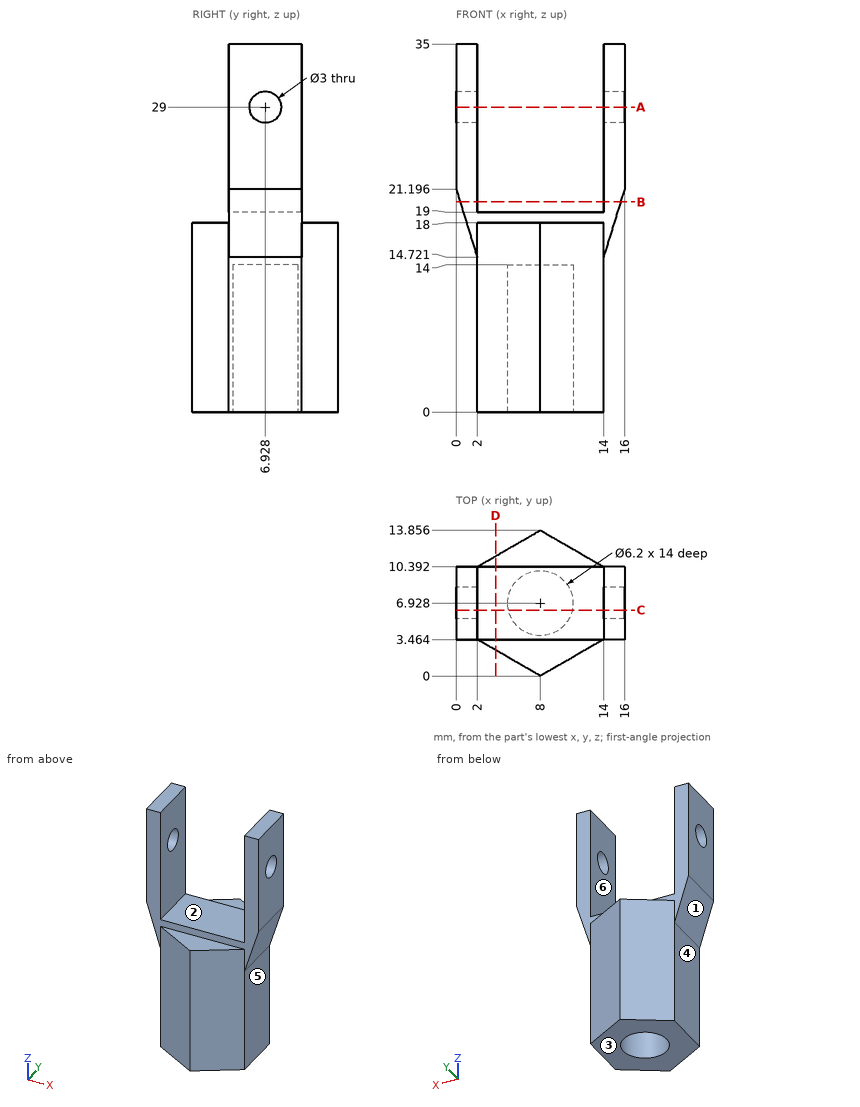
The drawing under review shows one solid part. Ordinate dimensions are in mm from its lowest x, y, z. A direction names the side the tool comes from. Coordinates: 2 decimals unless noted, no trailing zeros. Order: outer loops, then holes, each group sorted by start corner. A loop starts at its lowest first (then second) coordinate and runs counter-clockwise, first axis right, second up. Notation, with made-up numbers: (-39.75, -17) -> (13.25, -17) arc R20 ccw to (13.25, -9) -> close; hole circle Ø11 at (57.25, -35). An arc over 180 degrees is marked (long way). Answer as CSV lines item,"result".
Q1. For the marked faces 4, 5 and 6, list the 3-axis set-ups (+Z, -Z, +X, -X, +Y, -Y) from which the entire face can be reached by the end or side of a thin tool; tool diameter is ignored.
Model answer:
face 4,"-Z, -X, +Y, -Y"
face 5,"-Z, +X, +Y, -Y"
face 6,"+Z, +Y, -Y"
Q2. Draft analysis for pull direction X (two halves, no side actions). For the marked faces 1, 2 and 3, state which applies: released by +X, released by -X, zero draft, split by the parting line, or undercut.
Model answer:
face 1,"released by -X"
face 2,"undercut"
face 3,"zero draft"
Q3. We need section D-D (x = 3.75). State the section outline as (y, z) points.
Model answer:
outline,"(2.45, 0) -> (11.4, 0) -> (11.4, 18) -> (10.39, 18) -> (10.39, 19) -> (3.46, 19) -> (3.46, 18) -> (2.45, 18) -> close"
Q4. Wall thickness on line 1 along X through (y, z) = (5.75, 27.5); line 2 along Y through (x, z) = (14.7, 29); line 3 along Z through (x, y) = (2.75, 4.5): over which ranges is each line inside the solid? List them lowest first. Write a range as [from, to].
Model answer:
line 1,"x = [0, 2], [14, 16]"
line 2,"y = [3.46, 5.43], [8.43, 10.39]"
line 3,"z = [0, 19]"
Q5. We need section A-A (z = 29). State the section outline as (x, y) points, plus the area to 3 significant figures.
Model answer:
outline,"(0, 3.46) -> (2, 3.46) -> (2, 5.43) -> (0, 5.43) -> close; (0, 8.43) -> (2, 8.43) -> (2, 10.39) -> (0, 10.39) -> close; (14, 3.46) -> (16, 3.46) -> (16, 5.43) -> (14, 5.43) -> close; (14, 8.43) -> (16, 8.43) -> (16, 10.39) -> (14, 10.39) -> close"
area,"15.7 mm2"
Q6. We need section C-C (y = 6.25). State the section outline as (x, z) points (1 decimal).
Model answer:
outline,"(0, 21.2) -> (2, 14.7) -> (2, 0) -> (5, 0) -> (5, 14) -> (11, 14) -> (11, 0) -> (14, 0) -> (14, 14.7) -> (16, 21.2) -> (16, 27.7) -> (14, 27.7) -> (14, 19) -> (2, 19) -> (2, 27.7) -> (0, 27.7) -> close; (0, 30.3) -> (2, 30.3) -> (2, 35) -> (0, 35) -> close; (14, 30.3) -> (16, 30.3) -> (16, 35) -> (14, 35) -> close"
Q7. Clearance check with flat-ended pins moving along their axes: pin 1 Ø5 at (x, z) = (11.5, 21) entering from +Y; pin 2 Ø2 at (x, y) = (8.5, 10.5) entering from +Z; pin 3 Ø4 at (x, z) = (2.5, 12) entering from -Y. State where each tip first meets the part, or that it passes through.
Model answer:
pin 1,"stops at y = 10.39"
pin 2,"stops at z = 19"
pin 3,"stops at y = 2.02"
Q8. We need section B-B (z = 20). State the section outline as (x, y) points.
Model answer:
outline,"(0.37, 3.46) -> (2, 3.46) -> (2, 10.39) -> (0.37, 10.39) -> close; (14, 3.46) -> (15.63, 3.46) -> (15.63, 10.39) -> (14, 10.39) -> close"
